Autodesk Inventor part; units mm, degrees
ref_plane "YZ Plane" through (0, 0, 0) normal (1, 0, 0) x (0, 1, 0)
ref_plane "XZ Plane" through (0, 0, 0) normal (0, 1, 0) x (-1, 0, 0)
ref_plane "XY Plane" through (0, 0, 0) normal (0, 0, 1) x (1, 0, 0)
sketch "Sketch1" plane through (0, 0, 0) normal (0, 0, 1) x (1, 0, 0)
  circle A0 centre (0, 0) radius 12.5
  dimension "d0" = 25
extrude "Extrusion1" add sketch "Sketch1" against normal blind 290
sketch "Sketch2" plane through (0, 0, 0) normal (0, 0, 1) x (1, 0, 0)
  circle A0 centre (0, 0) radius 11
  dimension "d3" = 22
extrude "Extrusion2" add sketch "Sketch2" along normal blind 10
sketch "Sketch3" plane through (0, 0, 0) normal (0, 0, 1) x (1, 0, 0)
  circle A0 centre (0, 0) radius 8.5
  dimension "d6" = 17
extrude "Extrusion3" add sketch "Sketch3" along normal blind 45
sketch "Sketch4" plane through (0, 0, -290) normal (0, 0, -1) x (-1, 0, 0)
  circle A0 centre (0, 0) radius 11
  dimension "d9" = 22
extrude "Extrusion4" add sketch "Sketch4" along normal blind 10
sketch "Sketch5" plane through (0, 0, -300) normal (0, 0, -1) x (-1, 0, 0)
  circle A0 centre (0, 0) radius 8.5
  dimension "d12" = 17
extrude "Extrusion5" add sketch "Sketch5" along normal blind 35
The model under review builds one solid part; all positions refer to its coordinate system, in mm. A direction names the side the tool comes from. Coordinates: 2 decimals unless noted, no trailing zeros. Write each loop counter-clockwise with the first axis right and the second up, starting at its lowest first coordinate (ties: lowest second). Pieces come first, ordered by that corner, then holes. Notation, with made-up numbers: (34.25, 65) - (38.25, 65) arc R30 ccw to (38.25, 87) - close; hole circle Ø4 at (66.25, 83.25). An arc over 180 degrees is marked (long way). Answer in a Markdown table with one row per item. Add a question column.
Q1. For faces 1 (the face through (5, -10, 0)), 2 (the face through (2.38, 10.74, -294.93)), 3 (the face through (0, 0, 45)), list the 3-axis set-ups (+Z, -Z, +X, -X, +Y, -Y) from which the entire face can be reached by the end or side of a thin tool; tool diameter is ignored.
Q2. Clearance check with flat-ended pins moving along their axes: pin 1 (1.5 mm diameter, centred on y = 2.5, z = -38, fed in from -X); pin 2 (12 mm diameter, centred on x = 7, z = -15.5, fed in from -Y); pin 3 (1 mm diameter, centred on x = -9.5, y = -4.5, fed in from +Z). State where each tip first meets the part, or that it passes through.
Q3. Consider section A-A on x = 0. Give the boundary of the cut face in (y, z), then the cut area to 3 significant figures.
Q4. Consider section D-D on z = -305. Give the boundary of the cut face in (x, y).
Q5. Consider section C-C on z = -124. Give the boundary of the cut face in (x, y).
Q6. To check wall thickness, follow line 1 along Y through (x, z) = (-0.5, -221); line 2 along Z through (x, y) = (2.25, 10.25); line 3 along Z through (x, y) = (-9, -7.5). State the ranges of each line that lie inside material, in increasing order. Write a range as from..to.
Answers below:
| question | item | result |
|---|---|---|
| 1 | face 1 | +Z |
| 1 | face 2 | -Z |
| 1 | face 3 | +Z, +X, -X, +Y, -Y |
| 2 | pin 1 | x = -12.38 |
| 2 | pin 2 | y = -12.46 |
| 2 | pin 3 | z = 10 |
| 3 | outline | (-12.5, -290) - (-11, -290) - (-11, -300) - (-8.5, -300) - (-8.5, -335) - (8.5, -335) - (8.5, -300) - (11, -300) - (11, -290) - (12.5, -290) - (12.5, 0) - (11, 0) - (11, 10) - (8.5, 10) - (8.5, 45) - (-8.5, 45) - (-8.5, 10) - (-11, 10) - (-11, 0) - (-12.5, 0) - close |
| 3 | area | 8,880 mm² |
| 4 | outline | circle Ø17 at (0, 0) |
| 5 | outline | circle Ø25 at (0, 0) |
| 6 | line 1 | -12.49..12.49 |
| 6 | line 2 | -300..10 |
| 6 | line 3 | -290..0 |
